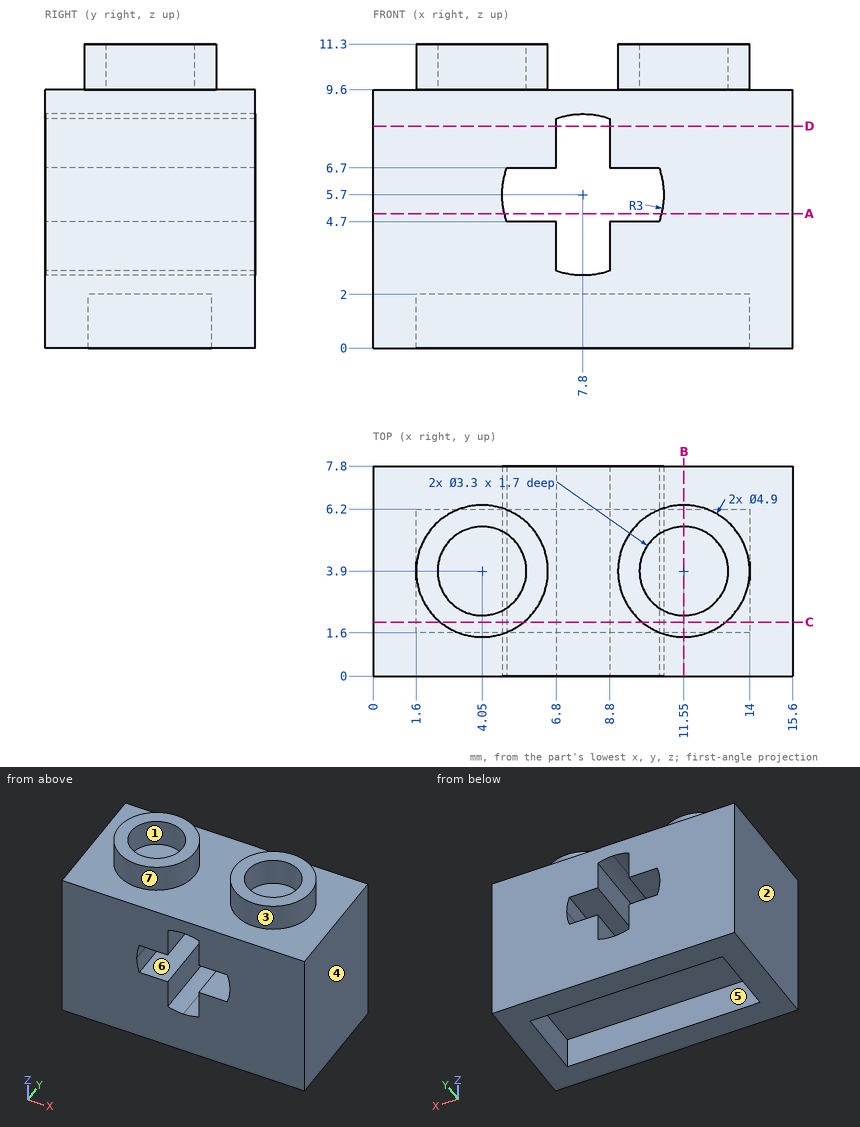
Geometry: see drawing. Coordinates: mm, zero at the bounding-box minimum. A direction names the side the tool comes from. Coordinates: 2 decimals unless noted, no trailing zeros. Write each loop counter-clockwise with the first axis right and the second up, starting at its lowest first coordinate (ties: lowest second). Pieces come first, ordered by that corner, then holes.
1) Set-up query: the marked faces 4, 5, 6 and 7. Return all of +Z, -Z, +X, -X, +Y, -Y with unobstructed straight access to the full face (end or side cutting, diameter ignored); none if empty.
2) Section A-A on z = 5. Output: boundary loops of the cut face in (x, y), and give its area (3 significant figures).
3) Mould query, pull axis Y, two halves, no side actions, for the marked faces 1, 2 and 3. Classes: pulls with the +Y half, pulls with the -Y half, needs draft (parallel to the pull), parting line crosses it, or undercut.
4) Section D-D on z = 8.25. Output: boundary loops of the cut face in (x, y), and give its area (3 significant figures).
5) Material intervals for line 1 along Y through (x, z) = (8.25, 1); line 2 along X through (y, z) = (7, 8.5); line 3 along Y through (x, z) = (11.55, 10.85), sorted ascending.
6) Pin query (flat end, axial travel): pin 1 Ø0.5 at (x, y) = (6, 4) entering from -Z; pin 2 Ø1.5 at (x, y) = (7.5, 5.5) entering from +Z. Return the tip coordinate at first contact, or that it passes through.
7) Section C-C on y = 2. Output: boundary loops of the cut face in (x, z), and give its area (3 significant figures).
8) Section B-B on x = 11.55. Output: boundary loops of the cut face in (y, z).
Check result:
1. face 4: +Z, -Z, +X, +Y, -Y
1. face 5: -Z
1. face 6: +Y, -Y
1. face 7: +Z
2. outline: (0, 0) - (4.88, 0) - (4.88, 7.8) - (0, 7.8) - close; (10.72, 0) - (15.6, 0) - (15.6, 7.8) - (10.72, 7.8) - close
2. area: 76.2 mm2
3. face 1: undercut
3. face 2: needs draft
3. face 3: parting line crosses it
4. outline: (0, 0) - (6.8, 0) - (6.8, 7.8) - (0, 7.8) - close; (8.8, 0) - (15.6, 0) - (15.6, 7.8) - (8.8, 7.8) - close
4. area: 106 mm2
5. line 1: y = 0 to 1.6, 6.2 to 7.8
5. line 2: x = 0 to 6.8, 8.8 to 15.6
5. line 3: y = 1.45 to 2.25, 5.55 to 6.35
6. pin 1: stops at z = 2
6. pin 2: stops at z = 9.6
7. outline: (0, 0) - (1.6, 0) - (1.6, 2) - (14, 2) - (14, 0) - (15.6, 0) - (15.6, 9.6) - (13.1, 9.6) - (13.1, 11.3) - (10, 11.3) - (10, 9.6) - (5.6, 9.6) - (5.6, 11.3) - (2.5, 11.3) - (2.5, 9.6) - (0, 9.6) - close; hole (4.97, 4.7) - (6.8, 4.7) - (6.8, 2.87) arc R3 ccw to (8.8, 2.87) - (8.8, 4.7) - (10.63, 4.7) arc R3 ccw to (10.63, 6.7) - (8.8, 6.7) - (8.8, 8.53) arc R3 ccw to (6.8, 8.53) - (6.8, 6.7) - (4.97, 6.7) arc R3 ccw to start
7. area: 116 mm2
8. outline: (0, 0) - (1.6, 0) - (1.6, 2) - (6.2, 2) - (6.2, 0) - (7.8, 0) - (7.8, 9.6) - (6.35, 9.6) - (6.35, 11.3) - (5.55, 11.3) - (5.55, 9.6) - (2.25, 9.6) - (2.25, 11.3) - (1.45, 11.3) - (1.45, 9.6) - (0, 9.6) - close
